```python
from build123d import *

# Parameters (mm, degrees)
ESQUISSE4_R             = 6.75
ENL_V_MAT_EXTRU_2_DEPTH = 224.575490607


with BuildPart() as part:
    # Esquisse1 → Révolution1 (revolve)
    with BuildSketch(Plane.XY, mode=Mode.PRIVATE) as r_volution1_sk:
        with BuildLine():
            Line((-155, 23), (-155, 32))
            Line((-155, 32), (-121, 32))
            Line((-121, 32), (-121, -12))
            Line((-121, -12), (-155, -12))
            Line((-155, -12), (-155, -3))
            Line((-155, -3), (-152, -3))
            Line((-152, -3), (-152, 0))
            Line((-152, 0), (-155, 0))
            Line((-155, 0), (-155, 7))
            ThreePointArc((-155, 7), (-150.094620701, 8.680407139), (-147.25, 13.015686517))
            ThreePointArc((-147.25, 13.015686517), (-145.5, 15), (-147.25, 16.984313483))
            ThreePointArc((-147.25, 16.984313483), (-150.094620701, 21.319592861), (-155, 23))
        make_face()
    revolve(r_volution1_sk.sketch.rotate(Axis((0, 44, 0), (0, -1, 0)), 270), axis=Axis((0, 44, 0), (0, -1, 0)))

    # Esquisse4 → Enlèv. mat.-Extru.2 (cut, through all)
    with BuildSketch(Plane(origin=(0, 32, 0), x_dir=(1, 0, 0), z_dir=(0, 1, 0))):
        with Locations(Location((-134, 0, 0), (0, 0, 270))):
            Circle(ESQUISSE4_R)
        with Locations(Location((-127.441573184, 41.408277246, 0), (0, 0, 270))):
            Circle(ESQUISSE4_R)
        with Locations(Location((-108.408277246, 78.763223807, 0), (0, 0, 270))):
            Circle(ESQUISSE4_R)
        with Locations(Location((-78.763223807, 108.408277246, 0), (0, 0, 270))):
            Circle(ESQUISSE4_R)
        with Locations(Location((-41.408277246, 127.441573184, 0), (0, 0, 270))):
            Circle(ESQUISSE4_R)
        with Locations(Location((0, 134, 0), (0, 0, 270))):
            Circle(ESQUISSE4_R)
        with Locations(Location((41.408277246, 127.441573184, 0), (0, 0, 270))):
            Circle(ESQUISSE4_R)
        with Locations(Location((78.763223807, 108.408277246, 0), (0, 0, 270))):
            Circle(ESQUISSE4_R)
        with Locations(Location((108.408277246, 78.763223807, 0), (0, 0, 270))):
            Circle(ESQUISSE4_R)
        with Locations(Location((127.441573184, 41.408277246, 0), (0, 0, 270))):
            Circle(ESQUISSE4_R)
        with Locations(Location((134, 0, 0), (0, 0, 270))):
            Circle(ESQUISSE4_R)
        with Locations(Location((127.441573184, -41.408277246, 0), (0, 0, 270))):
            Circle(ESQUISSE4_R)
        with Locations(Location((108.408277246, -78.763223807, 0), (0, 0, 270))):
            Circle(ESQUISSE4_R)
        with Locations(Location((78.763223807, -108.408277246, 0), (0, 0, 270))):
            Circle(ESQUISSE4_R)
        with Locations(Location((41.408277246, -127.441573184, 0), (0, 0, 270))):
            Circle(ESQUISSE4_R)
        with Locations(Location((0, -134, 0), (0, 0, 270))):
            Circle(ESQUISSE4_R)
        with Locations(Location((-41.408277246, -127.441573184, 0), (0, 0, 270))):
            Circle(ESQUISSE4_R)
        with Locations(Location((-78.763223807, -108.408277246, 0), (0, 0, 270))):
            Circle(ESQUISSE4_R)
        with Locations(Location((-108.408277246, -78.763223807, 0), (0, 0, 270))):
            Circle(ESQUISSE4_R)
        with Locations(Location((-127.441573184, -41.408277246, 0), (0, 0, 270))):
            Circle(ESQUISSE4_R)
    extrude(amount=-ENL_V_MAT_EXTRU_2_DEPTH, mode=Mode.SUBTRACT)


solid = part.part
```
Verification items for the finished model (mm, model axes). A direction names the side the tool comes from. Coordinates: 2 decimals unless noted, no trailing zeros. Answer as a JSON object with one key per item and string values. Group by question number.
(1) Material ranges on line 1 (X direction, y = 5, z = 0); line 2 (X direction, y = 6.5, z = 84); line 3 (Y direction, x = 100, z = 108), recorded low to high.
(2) Cross-section at A-A, the plane z = 0. State how many separate pieces and enclosed holes the cut face has, and give its area (3 significant figures).
(3) Tool access check on faces 1 (the face through (-47.397, 10.308, 130.556)), 2 (the face through (114, 0, -103)). Record the directions out of +Z, -Z, +X, -X, +Y, -Y that give a thin tool (end or side, any length) a straight path to the whole face; none if there is none.
(4) Gauge pin test, flat ends, axial feed: pin 1 (10 mm diameter, centred on x = 36.5, y = 23, fed in from -Z); pin 2 (10 mm diameter, centred on y = 2.5, z = 76.5, fed in from +X); pin 3 (4 mm diameter, centred on x = -28.5, y = 25.5, fed in from -Z). Record the tip position at first contact, or that the pin passes through.
(5) Release check for a two-part mould opening along X. For faces 3 (the face through (59.37, 3.55, 143.18)), 4 (the face through (91, -12, -80)), 5 (the face through (76.178, 10.308, 114.644)) record: +X half, -X half, draft (parallel to the pull), parting line (faces both ways), or undercut.
Reply:
{
 "1": {"line 1": "-155 to -140.75, -127.25 to -121, 121 to 127.25, 140.75 to 155", "line 2": "-130.27 to -112.67, -104.15 to -87.09, 87.09 to 104.15, 112.67 to 130.27", "line 3": "-12 to 13.02, 16.98 to 32"},
 "2": {"separate pieces": "4", "enclosed holes": "0", "area": "1,580 mm²"},
 "3": {"face 1": "+Y, -Y", "face 2": "none"},
 "4": {"pin 1": "z = -151.77", "pin 2": "x = 137.52", "pin 3": "z = -152.72"},
 "5": {"face 3": "parting line", "face 4": "draft", "face 5": "undercut"}
}
